```python
from build123d import *

# Parameters (mm, degrees)
F0_W     = 25
F0_H     = 70
F1_DEPTH = 2


with BuildPart() as f1:
    # F0 (on Top) → F1 (new body)
    with BuildSketch(Plane.XY):
        Rectangle(F0_W, F0_H)
        with BuildLine():
            Line((9, -32.591704), (-9, -32.591704))
            Line((-9, -32.591704), (-9, 8.219976))
            ThreePointArc((-9, 8.219976), (-8.985863, 8.724219), (-8.943498, 9.226878))
            ThreePointArc((-8.943498, 9.226878), (0.504243, 17.20584), (9, 8.219976))
            Line((9, 8.219976), (9, -32.591704))
        make_face(mode=Mode.SUBTRACT)
    extrude(amount=F1_DEPTH)


solid = f1.part
```
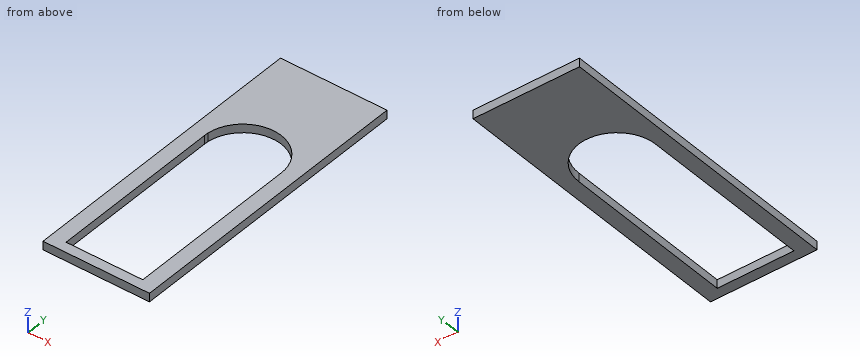
The listing builds one solid part. Answer for the finished solid, in the listing's coordinates (mm). Round coordinates to 2 decimals unless told otherwise and drop trailing zeros. Write each loop counter-clockwise with the first axis right and the second up, starting at its lowest first coordinate (ties: lowest second). Pieces come first, ordered by that corner, then holes. Notation, with made-up numbers: (60.25, 48) -> (94.25, 48) arc R17 cw to (94.25, 72) -> close; hole circle Ø4 at (-17.5, 67). An arc over 180 degrees is marked (long way). Write item = value, one per line.
1) Straight lines are drawn through the part: line 1 along X through (y, z) = (-19.5, 1.15); line 2 along Y through (x, z) = (-0.25, 1.9); line 3 along Y through (x, z) = (-3.5, 1.2). For each, find the intervals that lie inside material, in ascending order. Write a range as [from, to].
Check values:
line_1 = [-12.5, -9], [9, 12.5]
line_2 = [-35, -32.59], [17.22, 35]
line_3 = [-35, -32.59], [16.51, 35]
2) Section B-B on x = 0 is taken. Write down the section's boundary in (y, z), plus the area to 3 significant figures.
Check values:
outline = (-35, 0) -> (-32.59, 0) -> (-32.59, 2) -> (-35, 2) -> close; (17.22, 0) -> (35, 0) -> (35, 2) -> (17.22, 2) -> close
area = 40.4 mm²
3) Section A-A on y = -7.5 is taken. Write down the section's boundary in (x, z).
Check values:
outline = (-12.5, 0) -> (-9, 0) -> (-9, 2) -> (-12.5, 2) -> close; (9, 0) -> (12.5, 0) -> (12.5, 2) -> (9, 2) -> close
4) Given pin 1 (10 mm diameter, centred on x = 2, y = -0.5, fed in from +Z), flat-ended and moving along its own axis, determine where the tip first touches the part or whether it passes through.
Check values:
pin_1 = through
5) Section C-C on z = 0.85 is taken. Write down the section's boundary in (x, y), plus the area to 3 significant figures.
Check values:
outline = (-12.5, -35) -> (12.5, -35) -> (12.5, 35) -> (-12.5, 35) -> close; hole (-9, -32.59) -> (9, -32.59) -> (9, 8.22) arc R9 ccw to (-8.94, 9.23) arc R9 ccw to (-9, 8.22) -> close
area = 888 mm²
